Check sheet for the modelled part. Datum: model origin and axes. Units: mm. Face numbers are marked on the shaded views. A direction names the side the tool comes from. Coordinates: 2 decimals unless noted, no trailing zeros. Loops run counter-clockwise (first coordinate to the right, second up) from the corner with the lowest first, then second, coordinate; pieces in that order, holes last. Notation, with made-up numbers: M 48.25,5 L 53.25,5 A23 ccw 53.25,16 Z; hole C 14,17 d11. An arc over 180 degrees is marked long. Return JSON: item names as keys, results as strings.
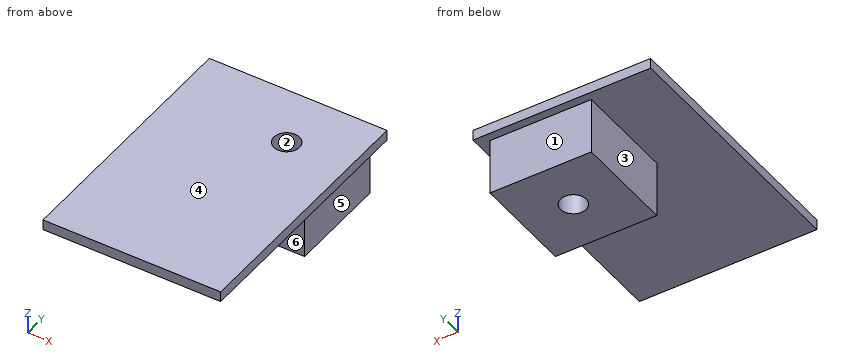
Autodesk Inventor part; units mm, degrees
ref_plane "YZ Plane" through (0, 0, 0) normal (1, 0, 0) x (0, 1, 0)
ref_plane "XZ Plane" through (0, 0, 0) normal (0, 1, 0) x (-1, 0, 0)
ref_plane "XY Plane" through (0, 0, 0) normal (0, 0, 1) x (1, 0, 0)
sketch "Skizze1" plane through (0, 0, 0) normal (0, 0, 1) x (1, 0, 0)
  line L0 (-4.85, 4.85) -> (4.85, 4.85)
  line L1 (4.85, 4.85) -> (4.85, -4.85)
  line L2 (4.85, -4.85) -> (-4.85, -4.85)
  line L3 (-4.85, -4.85) -> (-4.85, 4.85)
  line L4 (-4.85, 4.85) -> (4.85, -4.85) construction
  line L5 (4.85, 4.85) -> (-4.85, -4.85) construction
  circle A0 centre (0, 0) radius 1.2261
  dimension "d0" = 9.7
  dimension "d1" = 9.7
extrude "Extrusion1" add sketch "Skizze1" along normal blind 5.4
sketch "Sketch2" plane through (0, 0, 5.4) normal (0, 0, 1) x (1, 0, 0)
  circle A0 centre (0, 0) radius 1.2261
  line L0 (4.85, 4.85) -> (-4.85, 4.85)
  line L1 (-4.85, 4.85) -> (-4.85, -4.85)
  line L2 (-4.85, -4.85) -> (4.85, -4.85)
  line L3 (4.85, -4.85) -> (4.85, 4.85)
  line L4 (-11.05, 5.65) -> (5.95, 5.65)
  line L5 (5.95, 5.65) -> (5.95, -18.9856)
  line L6 (5.95, -18.9856) -> (-11.05, -18.9856)
  line L7 (-11.05, -18.9856) -> (-11.05, 5.65)
  dimension "d4" = 10.8
  dimension "d5" = 15.9
  dimension "d6" = 10.5
extrude "Extrusion2" add sketch "Sketch2" along normal blind 1 contours L3 L2 L1 L0 | L4 L5 L6 L7
properties part number "LG_G2_Lens"
1) Section check C-C on z = 1.75. Record the cut outline in (x, y).
Answers:
{"outline": "M -4.85,-4.85 L 4.85,-4.85 L 4.85,4.85 L -4.85,4.85 Z; hole C 0,0 d2.45"}
2) Go/stop test with flat-tipped pins: pin 1 Ø1.6 at (y, z) = (0, 3.5) entering from +X; pin 2 Ø1.5 at (x, y) = (0, 0) entering from -Z; pin 3 Ø2.5 at (y, z) = (-0.5, 3) entering from -X; pin 4 Ø2 at (x, z) = (-4.5, 1) entering from -Y. Record where each tip stops, or that it passes through.
Answers:
{"pin 1": "x = 4.85", "pin 2": "through", "pin 3": "x = -4.85", "pin 4": "y = -4.85"}
3) Section check B-B on x = 0. Record the cut outline in (y, z), then the cut area to 3 significant figures.
Answers:
{"outline": "M -18.99,5.4 L -4.85,5.4 L -4.85,0 L -1.23,0 L -1.23,6.4 L -18.99,6.4 Z; M 1.23,0 L 4.85,0 L 4.85,5.4 L 5.65,5.4 L 5.65,6.4 L 1.23,6.4 Z", "area": "61.3 mm²"}
4) Draft check along Y on the marked faces 1, 2 and 3. Enter one of: +Y half, -Y half, draft (parallel to the pull), parting line (faces both ways), or undercut.
Answers:
{"face 1": "+Y half", "face 2": "undercut", "face 3": "draft"}
5) Section check A-A on y = 0. Record the cut outline in (x, z), then the cut area to 3 significant figures.
Answers:
{"outline": "M -11.05,5.4 L -4.85,5.4 L -4.85,0 L -1.23,0 L -1.23,6.4 L -11.05,6.4 Z; M 1.23,0 L 4.85,0 L 4.85,5.4 L 5.95,5.4 L 5.95,6.4 L 1.23,6.4 Z", "area": "53.7 mm²"}
6) Set-up check for the marked faces 4, 5 and 6: record each of +Z, -Z, +X, -X, +Y, -Y from which the full face is reachable in a straight line by a thin tool's end or side.
Answers:
{"face 4": "+Z, +X, -X, +Y, -Y", "face 5": "-Z, +X, +Y, -Y", "face 6": "-Z, +X, -X, -Y"}
7) Scan lines: line 1 along Y through (x, z) = (0, 3); line 2 along Z through (x, y) = (-1.75, -15); line 3 along Y through (x, z) = (-0.5, 4). Record each from-to range of solid material in increasing order. Write a range as [from, to].
Answers:
{"line 1": "[-4.85, -1.23], [1.23, 4.85]", "line 2": "[5.4, 6.4]", "line 3": "[-4.85, -1.12], [1.12, 4.85]"}
8) Section check D-D on x = -2. Record the cut outline in (y, z), then the cut area to 3 significant figures.
Answers:
{"outline": "M -18.99,5.4 L -4.85,5.4 L -4.85,0 L 4.85,0 L 4.85,5.4 L 5.65,5.4 L 5.65,6.4 L -18.99,6.4 Z", "area": "77.0 mm²"}
